from build123d import *

# Parameters (mm, degrees)
SKETCH2_W           = 78.486
SKETCH2_H           = 56.896
BOSS_EXTRUDE1_DEPTH = 1.5875
SKETCH3_R           = 1.4605
CUT_EXTRUDE1_DEPTH  = 2.5875


with BuildPart() as part:
    # Sketch2 → Boss-Extrude1 (new body)
    with BuildSketch(Plane(origin=(0, 0, 0), x_dir=(1, 0, 0), z_dir=(0, 1, 0))):
        with Locations((39.243, 28.448)):
            Rectangle(SKETCH2_W, SKETCH2_H)
        Polygon((15.494, 39.878), (59.69, 39.878), (59.69, 36.83), (62.992, 36.83), (62.992, 20.066), (59.69, 20.066), (59.69, 17.018), (15.494, 17.018), (15.494, 20.066), (12.192, 20.066), (12.192, 36.83), (15.494, 36.83), align=None, mode=Mode.SUBTRACT)
    extrude(amount=BOSS_EXTRUDE1_DEPTH)

    # Sketch3 → Cut-Extrude1 (cut, through all)
    with BuildSketch(Plane(origin=(0, 1.5875, 0), x_dir=(1, 0, 0), z_dir=(0, 1, 0))):
        with Locations((6.35, 50.546)):
            Circle(SKETCH3_R)
        with Locations((6.35, 6.35)):
            Circle(SKETCH3_R)
        with Locations((72.136, 50.546)):
            Circle(SKETCH3_R)
        with Locations((72.136, 6.35)):
            Circle(SKETCH3_R)
    extrude(amount=-CUT_EXTRUDE1_DEPTH, mode=Mode.SUBTRACT)


solid = part.part
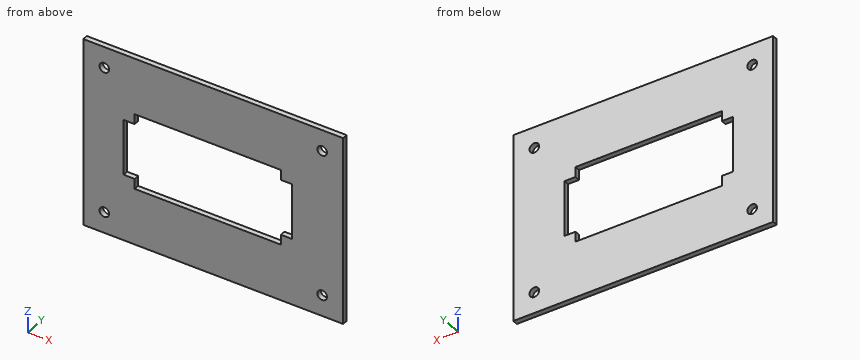
Read the model definition and answer for the solid it produces. Units are mm, in the model's axes. Coordinates: 2 decimals unless noted, no trailing zeros. Loops run counter-clockwise (first coordinate to the right, second up) from the corner with the lowest first, then second, coordinate; pieces in that order, holes last. Notation, with made-up numbers: (45.25, -31.5) -> (54.25, -31.5) arc R21 ccw to (54.25, -11.5) -> close; hole circle Ø7 at (22, 22). An arc over 180 degrees is marked (long way). Answer in a Markdown table with one row per item.
Item 1: A cutting plane is placed at A-A on x = 6.35. Determine the outline of the cut face in (y, z), plus the area to 3 significant figures.
Returned:
| item | result |
|---|---|
| outline | (0, -56.9) -> (1.59, -56.9) -> (1.59, -52.01) -> (0, -52.01) -> close; (0, -49.09) -> (1.59, -49.09) -> (1.59, -7.81) -> (0, -7.81) -> close; (0, -4.89) -> (1.59, -4.89) -> (1.59, 0) -> (0, 0) -> close |
| area | 81.0 mm^2 |
Item 2: A cutting plane is placed at C-C on x = 40. Determine the outline of the cut face in (y, z).
Returned:
| item | result |
|---|---|
| outline | (0, -56.9) -> (1.59, -56.9) -> (1.59, -39.88) -> (0, -39.88) -> close; (0, -17.02) -> (1.59, -17.02) -> (1.59, 0) -> (0, 0) -> close |
Item 3: Straight lines are drawn through the part: line 1 along X through (y, z) = (1.25, -6.35); line 2 along Z through (x, y) = (6.35, 0.6); line 3 along X through (y, z) = (1.2, -39). For each, find the intervals that lie inside material, in ascending order. Write a range as [from, to].
Returned:
| item | result |
|---|---|
| line 1 | x = [0, 4.89], [7.81, 70.68], [73.6, 78.49] |
| line 2 | z = [-56.9, -52.01], [-49.09, -7.81], [-4.89, 0] |
| line 3 | x = [0, 15.49], [59.69, 78.49] |
Item 4: A cutting plane is placed at B-B on z = -6.35. Determine the outline of the cut face in (x, y).
Returned:
| item | result |
|---|---|
| outline | (0, 0) -> (4.89, 0) -> (4.89, 1.59) -> (0, 1.59) -> close; (7.81, 0) -> (70.68, 0) -> (70.68, 1.59) -> (7.81, 1.59) -> close; (73.6, 0) -> (78.49, 0) -> (78.49, 1.59) -> (73.6, 1.59) -> close |
Item 5: This flat-tipped pin is pushed along its axis until it touches: P1, Ø2.5, axis at x = 6.35, z = -6.35, coming from the +Y side. Where does it stop, or does it pass through?
Returned:
| item | result |
|---|---|
| P1 | passes through |
Item 6: A cutting plane is placed at D-D on z = -28.5. Determine the outline of the cut face in (x, y), plus the area to 3 significant figures.
Returned:
| item | result |
|---|---|
| outline | (0, 0) -> (12.19, 0) -> (12.19, 1.59) -> (0, 1.59) -> close; (62.99, 0) -> (78.49, 0) -> (78.49, 1.59) -> (62.99, 1.59) -> close |
| area | 44.0 mm^2 |
